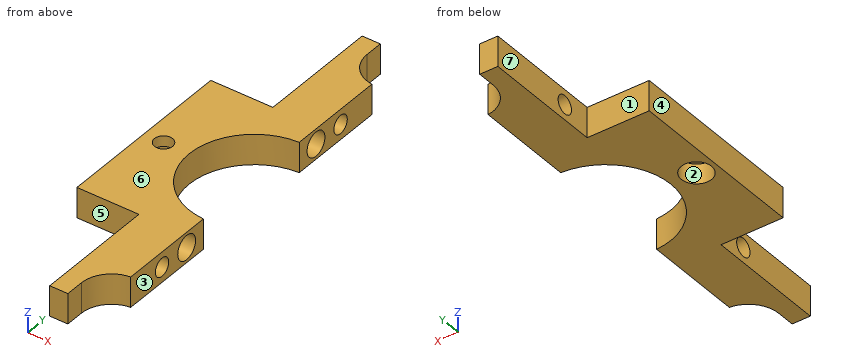
```python
from build123d import *

# Parameters (mm, degrees)
SKETCH1_R           = 3
EXTRUDE3_DEPTH      = 10
SKETCH6_R           = 5
CUT_EXTRUDE4_DEPTH  = 6.5
SKETCH7_R           = 3
CUT_EXTRUDE5_DEPTH  = 15
SKETCH9_R           = 3
CUT_EXTRUDE10_DEPTH = 15
SKETCH12_R          = 4
CUT_EXTRUDE13_DEPTH = 10


with BuildPart() as part:
    # Sketch1 → Extrude3 (new body)
    with BuildSketch(Plane.XY):
        with BuildLine():
            Line((26.5, 134), (26.5, 140))
            Line((26.5, 140), (20.5, 140))
            Line((20.5, 140), (20.5, 100))
            Line((20.5, 100), (5.5, 100))
            Line((5.5, 100), (0, 100))
            Line((0, 100), (0, 40))
            Line((0, 40), (5.5, 40))
            Line((5.5, 40), (20.5, 40))
            Line((20.5, 40), (20.5, 0))
            Line((20.5, 0), (26.5, 0))
            Line((26.5, 0), (26.5, 6))
            ThreePointArc((26.5, 6), (29.083801513, 12.708203932), (35.5, 15.949874371))
            Line((35.5, 15.949874371), (35.5, 40))
            Line((35.5, 40), (35.5, 48.523268405))
            ThreePointArc((35.5, 48.523268405), (15, 70), (35.5, 91.476731595))
            Line((35.5, 91.476731595), (35.5, 100))
            Line((35.5, 100), (35.5, 124.050125629))
            ThreePointArc((35.5, 124.050125629), (29.083801513, 127.291796068), (26.5, 134))
        make_face()
        with Locations((6.5, 70)):
            Circle(SKETCH1_R, mode=Mode.SUBTRACT)
    extrude(amount=EXTRUDE3_DEPTH)

    # Sketch6 → Cut-Extrude4 (cut)
    with BuildSketch(Plane(origin=(0, 0, 0), x_dir=(-1, 0, 0), z_dir=(0, 0, -1))):
        with Locations((-6.5, 70)):
            Circle(SKETCH6_R)
    extrude(amount=-CUT_EXTRUDE4_DEPTH, mode=Mode.SUBTRACT)

    # Sketch7 → Cut-Extrude5 (cut)
    with BuildSketch(Plane.ZY.offset(-20.5)):
        with Locations((5, 30)):
            Circle(SKETCH7_R)
    extrude(amount=-CUT_EXTRUDE5_DEPTH, mode=Mode.SUBTRACT)

    # Sketch9 → Cut-Extrude10 (cut)
    with BuildSketch(Plane.ZY.offset(-20.5)):
        with Locations((5, 110)):
            Circle(SKETCH9_R)
    extrude(amount=-CUT_EXTRUDE10_DEPTH, mode=Mode.SUBTRACT)

    # Sketch12 → Cut-Extrude13 (cut)
    with BuildSketch(Plane(origin=(35.5, 0, 0), x_dir=(0, 0, -1), z_dir=(1, 0, 0))):
        with Locations((-5, 98.976731595)):
            Circle(SKETCH12_R)
        with Locations((-5, 41.023268405)):
            Circle(SKETCH12_R)
    extrude(amount=-CUT_EXTRUDE13_DEPTH, mode=Mode.SUBTRACT)


solid = part.part
```
For this review, take the finished solid that the model builds, in its own axes (mm). Face numbers are marked on the shaded views. A direction names the side the tool comes from. Coordinates: 2 decimals unless noted, no trailing zeros. Order: outer loops, then holes, each group sorted by start corner. A loop starts at its lowest first (then second) coordinate and runs counter-clockwise, first axis right, second up. Notation, with made-up numbers: (73.25, 48.5) - (114.25, 48.5) arc R28 cw to (114.25, 81.5) - close; hole circle Ø8 at (29.25, -26). An arc over 180 degrees is marked (long way). Answer as a JSON object with one key per item and string values. Group by question number.
1. The part is to be moulded in two halves that separate along X. For the marked faces 1, 2, 3 and 4, say which applies: pulls with the +X half, pulls with the -X half, needs draft (parallel to the pull), parting line crosses it, or undercut.
2. We need section B-B on y = 110. State the section outline as (x, z) points, then the cut area to 3 significant figures.
3. Clearance check with flat-ended pins moving along their axes: P1, Ø1, axis at y = 57.5, z = 3.5, coming from the +X side; P2, Ø3, axis at y = 15.5, z = 5, coming from the -X side; P3, Ø4, axis at x = 11.5, z = 5, coming from the +Y side. State where each tip first meets the part, or that it passes through.
4. We need section A-A on z = 5. Give the number of separate pieces and of enclosed holes in the cut face, then the cut area to 3 significant figures.
5. For probe 1 along Y at (x, z) = (6.5, 8.7); probe 2 along Y at (x, z) = (7, 2); probe 3 along X at (y, z) = (70, 7.8), list the stretches that pass through material, from the lowest coordinate up.
6. For the marked faces 5, 6 and 7, list the 3-axis set-ups (+Z, -Z, +X, -X, +Y, -Y) from which the entire face can be reached by the end or side of a thin tool; tool diameter is ignored.
7. We need section D-D on x = 6.5. State the section outline as (y, z) points.
8. We need section C-C on x = 31.5. State the section outline as (y, z) points, then the cut area to 3 significant figures.
Final values:
{
 "1": {"face 1": "needs draft", "face 2": "undercut", "face 3": "pulls with the +X half", "face 4": "pulls with the -X half"},
 "2": {"outline": "(20.5, 0) - (35.5, 0) - (35.5, 2) - (20.5, 2) - close; (20.5, 8) - (35.5, 8) - (35.5, 10) - (20.5, 10) - close", "area": "60.0 mm²"},
 "3": {"P1": "x = 19.38", "P2": "x = 20.5", "P3": "y = 100"},
 "4": {"separate pieces": "3", "enclosed holes": "1", "area": "1,980 mm²"},
 "5": {"probe 1": "40 to 67, 73 to 100", "probe 2": "40 to 65.03, 74.97 to 100", "probe 3": "0 to 3.5, 9.5 to 15"},
 "6": {"face 5": "+Z, -Z, -X, -Y", "face 6": "+Z, +X, -X, +Y, -Y", "face 7": "+Z, -Z, -X, +Y"},
 "7": {"outline": "(40, 0) - (65, 0) - (65, 6.5) - (67, 6.5) - (67, 10) - (40, 10) - close; (73, 6.5) - (75, 6.5) - (75, 0) - (100, 0) - (100, 10) - (73, 10) - close"},
 "8": {"outline": "(14.66, 0) - (49.09, 0) - (49.09, 10) - (14.66, 10) - close; (90.91, 0) - (125.34, 0) - (125.34, 10) - (90.91, 10) - close; hole circle Ø6 at (30, 5); hole circle Ø8 at (41.02, 5); hole circle Ø8 at (98.98, 5); hole circle Ø6 at (110, 5)", "area": "532 mm²"}
}
